```python
from build123d import *

# Parameters (mm, degrees)
F0_W      = 28.448
F0_H      = 60.96
F1_DEPTH  = 48.26
F2_W      = 25.4
F2_H      = 10.16
F3_DEPTH  = 28.449
F4_W      = 14.224
F4_H      = 39.37
F5_DEPTH  = 48.261
F6_W      = 35.56
F6_H      = 28.448
F7_DEPTH  = 90.932
F8_W      = 19.304
F8_H      = 11.176
F9_DEPTH  = 48.261
F11_DEPTH = 48.261
F12_R     = 6.35
F13_DEPTH = 48.261


with BuildPart() as f1:
    # F0 (on Top) → F1 (new body)
    with BuildSketch(Plane.XY):
        Rectangle(F0_W, F0_H)
    extrude(amount=F1_DEPTH)

    # F2 (on face) → F3 (cut, through all)
    with BuildSketch(Plane.YZ.offset(14.224)):
        with Locations((0, 43.18)):
            Rectangle(F2_W, F2_H)
    extrude(amount=-F3_DEPTH, mode=Mode.SUBTRACT)

    # F4 (on face) → F5 (cut, through all)
    with BuildSketch(Plane.XY.offset(48.26)):
        with Locations((-7.112, -1.905)):
            Rectangle(F4_W, F4_H)
    extrude(amount=-F5_DEPTH, mode=Mode.SUBTRACT)

    # F6 (on face) → F7 (join)
    with BuildSketch(Plane.YZ.offset(14.224)):
        with Locations((0, 14.224)):
            Rectangle(F6_W, F6_H)
    extrude(amount=F7_DEPTH)

    # F8 (on face) → F9 (cut, through all)
    with BuildSketch(Plane.XZ.offset(17.78)):
        with Locations((95.504, 22.86)):
            Rectangle(F8_W, F8_H)
    extrude(amount=-F9_DEPTH, mode=Mode.SUBTRACT)

    # F10 (on face) → F11 (cut, through all)
    with BuildSketch(Plane(origin=(0, 0, 0), x_dir=(1, 0, 0), z_dir=(0, 0, -1))):
        Polygon((74.360137, 17.78), (105.156, 0), (105.156, 17.78), align=None)
        Polygon((105.156, -17.78), (105.156, 0), (74.360137, -17.78), align=None)
    extrude(amount=-F11_DEPTH, mode=Mode.SUBTRACT)

    # F12 (on face) → F13 (cut, through all)
    with BuildSketch(Plane.XZ.offset(17.78)):
        with Locations((49.276, 14.224)):
            Circle(F12_R)
    extrude(amount=-F13_DEPTH, mode=Mode.SUBTRACT)


solid = f1.part
```
CAD build for the part. Positions are in the model's coordinates, mm. A direction names the side the tool comes from. Give positions to 0.01 mm unless a question says otherwise; leave off trailing zeros. Order: outer loops, then holes, each group sorted by start corner. A loop starts at its lowest first (then second) coordinate and runs counter-clockwise, first axis right, second up.
(1) Saw through at B-B, the plane x = 8. Give the cut face in (y, z), then the cut area to 3 significant figures.
(2) Tool access for faces 4 (the flat face through (44, 17.78, 8)), 5 (the flat face through (85.852, 0, 23)), 6 (the flat face through (7, 12.7, 43)), 7 (the flat face through (-7, -21.59, 24)): list every direction of +Z, -Z, +X, -X, +Y, -Y with a clear straight run to the whole face (end or side of a thin tool).
(3) Drill centre lines: L1, parallel to Y at x = -7, z = 22; L2, parallel to Z at x = 12, y = -5.5; L3, parallel to X at y = -13, z = 32.5. Where is each one in solid material? Low to high.
(4) Mould opens along X. For faces 1 (the flat face through (7, 0, 38.1)), 2 (the cylindrical face through (55.333, -0.249, 16.131)), 3 (the flat face through (-14.224, -26, 24)) say: released by +X, released by -X, zero draft, split by the parting line, or undercut.
(5) Saw through at D-D, the plane y = 7.5. Give the cut face in (x, z), then the cut area to 3 significant figures.
(6) Saw through at A-A, the plane z = 43.5. Give the cut face in (x, y), then the cut area to 3 significant figures.
(7) Flat gauge pins, fed straight in: pin 1 (8.5 mm diameter, centred on x = 53.5, z = 9.5, fed in from -Y); pin 2 (21 mm diameter, centred on x = 97, y = 4, fed in from +Z); pin 3 (10 mm diameter, centred on x = 69, y = -18, fed in from +Z). Where does each tip first touch, or does it go through?
(8) Saw through at C-C, the plane z = 34.5. Give the cut face in (x, y).
Results found:
1. outline: (-30.48, 0) - (30.48, 0) - (30.48, 48.26) - (12.7, 48.26) - (12.7, 38.1) - (-12.7, 38.1) - (-12.7, 48.26) - (-30.48, 48.26) - close
1. area: 2,680 mm2
2. face 4: +Z, -Z, +X, +Y
2. face 5: +Z, +X, +Y, -Y
2. face 6: +Z, +X, -X
2. face 7: +Z, -Z, -X
3. L1: y = -30.48 to -21.59, 17.78 to 30.48
3. L2: z = 0 to 38.1
3. L3: x = 0 to 14.22
4. face 1: zero draft
4. face 2: undercut
4. face 3: released by -X
5. outline: (0, 0) - (92.17, 0) - (92.17, 17.27) - (85.85, 17.27) - (85.85, 28.45) - (14.22, 28.45) - (14.22, 38.1) - (0, 38.1) - close; hole circle Ø12.7 at (49.28, 14.22)
5. area: 2,560 mm2
6. outline: (-14.22, -30.48) - (14.22, -30.48) - (14.22, -12.7) - (0, -12.7) - (0, -21.59) - (-14.22, -21.59) - close; (-14.22, 17.78) - (0, 17.78) - (0, 12.7) - (14.22, 12.7) - (14.22, 30.48) - (-14.22, 30.48) - close
6. area: 813 mm2
7. pin 1: stops at y = -17.78
7. pin 2: stops at z = 17.27
7. pin 3: stops at z = 28.45
8. outline: (-14.22, -30.48) - (14.22, -30.48) - (14.22, 30.48) - (-14.22, 30.48) - (-14.22, 17.78) - (0, 17.78) - (0, -21.59) - (-14.22, -21.59) - close
